from build123d import *

# Parameters (mm, degrees)
BOSS_EXTRUDE1_DEPTH      = 7.5
BOSS_EXTRUDE1_DEPTH_BACK = 7.5
SKETCH3_W                = 200
SKETCH3_H                = 15
CUT_EXTRUDE1_DEPTH       = 101.560926806
FILLET1_R                = 0.503257554
LPATTERN1_COUNT          = 42
LPATTERN1_PITCH          = 4.71238898
FILLET1_OF_LPATTERN1_R   = 0.503257554
CUT_EXTRUDE2_DEPTH       = 101.560926806
CUT_EXTRUDE2_DEPTH_BACK  = 101.560926806
SKETCH5_W                = 4.71238898
SKETCH5_H                = 3.375
CUT_EXTRUDE3_DEPTH       = 101.560926806
CUT_EXTRUDE3_DEPTH_BACK  = 101.560926806
SKETCH6_W                = 13.890612777
SKETCH6_H                = 21.950597968
CUT_EXTRUDE6_DEPTH       = 101.560926806
CUT_EXTRUDE6_DEPTH_BACK  = 101.560926806
SKETCH8_W                = 175.100830171
SKETCH8_H                = 44.946806771
SKETCH9_W                = 55.501850732
SKETCH9_H                = 10.784038355
CUT_EXTRUDE7_DEPTH       = 101.560926806
SKETCH10_W               = 10
SKETCH10_H               = 38
BOSS_EXTRUDE2_DEPTH      = 6.9
SKETCH11_W               = 12.54
SKETCH11_H               = 38
BOSS_EXTRUDE3_DEPTH      = 50
SKETCH12_W               = 2.54
SKETCH12_H               = 35
CUT_EXTRUDE8_DEPTH       = 121.701325593
CHAMFER1_SIZE            = 3
CHAMFER1_SIZE2           = 1.816762814
FILLET2_R                = 10
SKETCH13_W               = 39.144192087
SKETCH13_H               = 30
CUT_EXTRUDE9_DEPTH       = 5
CHAMFER2_SIZE            = 2
SKETCH14_R               = 1.5
CUT_EXTRUDE10_DEPTH      = 78.944675893


with BuildPart() as part:
    # Sketch3 → Boss-Extrude1 (new, two sides: drawn at the far end of the back side and taken through both)
    with BuildSketch(Plane.XY.offset(-BOSS_EXTRUDE1_DEPTH_BACK)):
        Rectangle(SKETCH3_W, SKETCH3_H)
    extrude(amount=BOSS_EXTRUDE1_DEPTH + BOSS_EXTRUDE1_DEPTH_BACK)

    # Sketch4 → Cut-Extrude1 (cut, symmetric)
    with BuildSketch(Plane.XY):
        Polygon((-94.247779608, 7.5), (-94.247779608, 4.125), (-94.743432664, 4.125), (-95.971832204, 7.5), align=None)
        Polygon((-97.236115992, 7.5), (-98.464515532, 4.125), (-98.960168588, 4.125), (-98.960168588, 7.5), align=None)
    cut_extrude1 = extrude(amount=CUT_EXTRUDE1_DEPTH, both=True, mode=Mode.SUBTRACT)

    # Fillet1
    fillet1_edges = [part.edges().sort_by_distance(p)[0] for p in [
        (-95.971832204, 7.5, 0),
        (-94.743432664, 4.125, 0),
        (-97.236115992, 7.5, 0),
        (-98.464515532, 4.125, 0),
    ]]
    fillet(fillet1_edges, radius=FILLET1_R)

    # LPattern1: Cut-Extrude1 ×42
    with Locations(*[(i * LPATTERN1_PITCH, 0, 0) for i in range(1, LPATTERN1_COUNT)]):
        add(cut_extrude1, mode=Mode.SUBTRACT)

    # Fillet1 of LPattern1
    fillet1_of_lpattern1_edges = [part.edges().sort_by_distance(p)[0] for p in [
        (-91.259443224, 7.5, 0),
        (-90.031043683, 4.125, 0),
        (-92.523727011, 7.5, 0),
        (-93.752126552, 4.125, 0),
        (-86.547054243, 7.5, 0),
        (-85.318654703, 4.125, 0),
        (-87.811338031, 7.5, 0),
        (-89.039737571, 4.125, 0),
        (-81.834665263, 7.5, 0),
        (-80.606265722, 4.125, 0),
        (-83.09894905, 7.5, 0),
        (-84.327348591, 4.125, 0),
        (-77.122276283, 7.5, 0),
        (-75.893876742, 4.125, 0),
        (-78.38656007, 7.5, 0),
        (-79.614959611, 4.125, 0),
        (-72.409887302, 7.5, 0),
        (-71.181487762, 4.125, 0),
        (-73.67417109, 7.5, 0),
        (-74.90257063, 4.125, 0),
        (-67.697498322, 7.5, 0),
        (-66.469098781, 4.125, 0),
        (-68.961782109, 7.5, 0),
        (-70.19018165, 4.125, 0),
        (-62.985109342, 7.5, 0),
        (-61.756709801, 4.125, 0),
        (-64.249393129, 7.5, 0),
        (-65.47779267, 4.125, 0),
        (-58.272720361, 7.5, 0),
        (-57.04432082, 4.125, 0),
        (-59.537004149, 7.5, 0),
        (-60.765403689, 4.125, 0),
        (-53.560331381, 7.5, 0),
        (-52.33193184, 4.125, 0),
        (-54.824615168, 7.5, 0),
        (-56.053014709, 4.125, 0),
        (-48.8479424, 7.5, 0),
        (-47.61954286, 4.125, 0),
        (-50.112226188, 7.5, 0),
        (-51.340625728, 4.125, 0),
        (-44.13555342, 7.5, 0),
        (-42.907153879, 4.125, 0),
        (-45.399837207, 7.5, 0),
        (-46.628236748, 4.125, 0),
        (-39.42316444, 7.5, 0),
        (-38.194764899, 4.125, 0),
        (-40.687448227, 7.5, 0),
        (-41.915847768, 4.125, 0),
        (-34.710775459, 7.5, 0),
        (-33.482375919, 4.125, 0),
        (-35.975059247, 7.5, 0),
        (-37.203458787, 4.125, 0),
        (-29.998386479, 7.5, 0),
        (-28.769986938, 4.125, 0),
        (-31.262670266, 7.5, 0),
        (-32.491069807, 4.125, 0),
        (-25.285997498, 7.5, 0),
        (-24.057597958, 4.125, 0),
        (-26.550281286, 7.5, 0),
        (-27.778680826, 4.125, 0),
        (-20.573608518, 7.5, 0),
        (-19.345208977, 4.125, 0),
        (-21.837892305, 7.5, 0),
        (-23.066291846, 4.125, 0),
        (-15.861219538, 7.5, 0),
        (-14.632819997, 4.125, 0),
        (-17.125503325, 7.5, 0),
        (-18.353902866, 4.125, 0),
        (-11.148830557, 7.5, 0),
        (-9.920431017, 4.125, 0),
        (-12.413114345, 7.5, 0),
        (-13.641513885, 4.125, 0),
        (-6.436441577, 7.5, 0),
        (-5.208042036, 4.125, 0),
        (-7.700725364, 7.5, 0),
        (-8.929124905, 4.125, 0),
        (-1.724052597, 7.5, 0),
        (-0.495653056, 4.125, 0),
        (-2.988336384, 7.5, 0),
        (-4.216735925, 4.125, 0),
        (2.988336384, 7.5, 0),
        (4.216735925, 4.125, 0),
        (1.724052596, 7.5, 0),
        (0.495653056, 4.125, 0),
        (7.700725364, 7.5, 0),
        (8.929124905, 4.125, 0),
        (6.436441577, 7.5, 0),
        (5.208042036, 4.125, 0),
        (12.413114345, 7.5, 0),
        (13.641513885, 4.125, 0),
        (11.148830557, 7.5, 0),
        (9.920431017, 4.125, 0),
        (17.125503325, 7.5, 0),
        (18.353902866, 4.125, 0),
        (15.861219538, 7.5, 0),
        (14.632819997, 4.125, 0),
        (21.837892305, 7.5, 0),
        (23.066291846, 4.125, 0),
        (20.573608518, 7.5, 0),
        (19.345208977, 4.125, 0),
        (26.550281286, 7.5, 0),
        (27.778680826, 4.125, 0),
        (25.285997498, 7.5, 0),
        (24.057597958, 4.125, 0),
        (31.262670266, 7.5, 0),
        (32.491069807, 4.125, 0),
        (29.998386479, 7.5, 0),
        (28.769986938, 4.125, 0),
        (35.975059247, 7.5, 0),
        (37.203458787, 4.125, 0),
        (34.710775459, 7.5, 0),
        (33.482375919, 4.125, 0),
        (40.687448227, 7.5, 0),
        (41.915847768, 4.125, 0),
        (39.42316444, 7.5, 0),
        (38.194764899, 4.125, 0),
        (45.399837207, 7.5, 0),
        (46.628236748, 4.125, 0),
        (44.13555342, 7.5, 0),
        (42.907153879, 4.125, 0),
        (50.112226188, 7.5, 0),
        (51.340625728, 4.125, 0),
        (48.8479424, 7.5, 0),
        (47.61954286, 4.125, 0),
        (54.824615168, 7.5, 0),
        (56.053014709, 4.125, 0),
        (53.560331381, 7.5, 0),
        (52.33193184, 4.125, 0),
        (59.537004148, 7.5, 0),
        (60.765403689, 4.125, 0),
        (58.272720361, 7.5, 0),
        (57.04432082, 4.125, 0),
        (64.249393129, 7.5, 0),
        (65.47779267, 4.125, 0),
        (62.985109341, 7.5, 0),
        (61.756709801, 4.125, 0),
        (68.961782109, 7.5, 0),
        (70.19018165, 4.125, 0),
        (67.697498322, 7.5, 0),
        (66.469098781, 4.125, 0),
        (73.67417109, 7.5, 0),
        (74.90257063, 4.125, 0),
        (72.409887302, 7.5, 0),
        (71.181487762, 4.125, 0),
        (78.38656007, 7.5, 0),
        (79.614959611, 4.125, 0),
        (77.122276283, 7.5, 0),
        (75.893876742, 4.125, 0),
        (83.09894905, 7.5, 0),
        (84.327348591, 4.125, 0),
        (81.834665263, 7.5, 0),
        (80.606265722, 4.125, 0),
        (87.811338031, 7.5, 0),
        (89.039737571, 4.125, 0),
        (86.547054243, 7.5, 0),
        (85.318654703, 4.125, 0),
        (92.523727011, 7.5, 0),
        (93.752126552, 4.125, 0),
        (91.259443224, 7.5, 0),
        (90.031043683, 4.125, 0),
        (97.236115992, 7.5, 0),
        (98.464515532, 4.125, 0),
        (95.971832204, 7.5, 0),
        (94.743432664, 4.125, 0),
    ]]
    fillet(fillet1_of_lpattern1_edges, radius=FILLET1_OF_LPATTERN1_R)

    # Sketch5 → Cut-Extrude2 (cut, two sides: drawn at the far end of the back side and taken through both)
    with BuildSketch(Plane.XY.offset(-CUT_EXTRUDE2_DEPTH_BACK)):
        with Locations((-101.316363078, 5.8125)):
            Rectangle(SKETCH5_W, SKETCH5_H)
        with Locations((101.316363078, 5.8125)):
            Rectangle(SKETCH5_W, SKETCH5_H)
    extrude(amount=CUT_EXTRUDE2_DEPTH + CUT_EXTRUDE2_DEPTH_BACK, mode=Mode.SUBTRACT)

    # Sketch6 → Cut-Extrude3 (cut, two sides: drawn at the far end of the back side and taken through both)
    with BuildSketch(Plane(origin=(0, 0, 0), x_dir=(0, 0, -1), z_dir=(1, 0, 0)).offset(-CUT_EXTRUDE3_DEPTH_BACK)):
        with Locations((5.945306389, -0.750264579)):
            Rectangle(SKETCH6_W, SKETCH6_H)
    extrude(amount=CUT_EXTRUDE3_DEPTH + CUT_EXTRUDE3_DEPTH_BACK, mode=Mode.SUBTRACT)

    # Sketch8 → Cut-Extrude6 (cut, two sides: drawn at the far end of the back side and taken through both)
    with BuildSketch(Plane.XY.offset(-CUT_EXTRUDE6_DEPTH_BACK)):
        with Locations((27.550415086, 7.242613414)):
            Rectangle(SKETCH8_W, SKETCH8_H)
    extrude(amount=CUT_EXTRUDE6_DEPTH + CUT_EXTRUDE6_DEPTH_BACK, mode=Mode.SUBTRACT)

    # Sketch9 → Cut-Extrude7 (cut, through all)
    with BuildSketch(Plane.XY):
        with Locations((-76.828993169, -6.642019178)):
            Rectangle(SKETCH9_W, SKETCH9_H)
    extrude(amount=CUT_EXTRUDE7_DEPTH, mode=Mode.SUBTRACT)

    # Sketch10 → Boss-Extrude2 (add)
    with BuildSketch(Plane(origin=(0, 0, 1), x_dir=(-1, 0, 0), z_dir=(0, 0, -1))):
        with Locations((65, 17.75)):
            Rectangle(SKETCH10_W, SKETCH10_H)
    extrude(amount=BOSS_EXTRUDE2_DEPTH)

    # Sketch11 → Boss-Extrude3 (add)
    with BuildSketch(Plane(origin=(0, 0, -5.9), x_dir=(-1, 0, 0), z_dir=(0, 0, -1))):
        with Locations((66.27, 17.75)):
            Rectangle(SKETCH11_W, SKETCH11_H)
    extrude(amount=BOSS_EXTRUDE3_DEPTH)

    # Sketch12 → Cut-Extrude8 (cut, through all)
    with BuildSketch(Plane.XZ.offset(1.25)):
        with Locations((-71.27, -23.4)):
            Rectangle(SKETCH12_W, SKETCH12_H)
        Polygon((-60, -5.9), (-63.8, -55.9), (-60, -55.9), align=None)
    extrude(amount=-CUT_EXTRUDE8_DEPTH, mode=Mode.SUBTRACT)

    # Chamfer1
    chamfer1_edges = [part.edges().sort_by_distance(p)[0] for p in [
        (-63.8, 17.75, -55.9),
    ]]
    chamfer1_side = [part.faces().sort_by_distance(p)[0] for p in [
        (-61.9, 17.75, -30.9),
    ]]
    chamfer(chamfer1_edges, length=CHAMFER1_SIZE, length2=CHAMFER1_SIZE2, reference=chamfer1_side[0])

    # Fillet2
    # the kernel refuses this fillet: 10 mm, written as the material it adds along each edge
    with BuildSketch(Plane(origin=(-70, -1.25, -40.9), x_dir=(-1, 0, 0), z_dir=(0, 1, 0))) as fillet2_piece_1:
        with BuildLine():
            CenterArc((10, 6.659459438), FILLET2_R, 180, 41.754936598)
            Line((0, 6.659459438), (-0.2, 6.659459438))
            Line((-0.2, 6.659459438), (-0.2, 0))
            Line((-0.2, 0), (0, -0.2))
            ThreePointArc((0, -0.2), (1.27, -0.2), (2.3908, -0.133189189))
            Line((2.3908, -0.133189189), (2.54, 0))
        make_face()
    extrude(amount=38)

    # Sketch13 → Cut-Extrude9 (cut)
    with BuildSketch(Plane(origin=(-59.20960532, 0, 4.499930004), x_dir=(-0.07578145826840343, 0, -0.997124450900044), z_dir=(0.997124450900044, 0, -0.07578145826840343))):
        with Locations((34.0020178, 17.75)):
            Rectangle(SKETCH13_W, SKETCH13_H)
    extrude(amount=-CUT_EXTRUDE9_DEPTH, mode=Mode.SUBTRACT)

    # Chamfer2
    chamfer2_edges = [part.edges().sort_by_distance(p)[0] for p in [
        (-62.79593696, 2.75, -9.699044158),
        (-62.79593696, 32.75, -9.699044158),
        (-65.762340919, 32.75, -48.730675198),
        (-65.762340919, 2.75, -48.730675198),
    ]]
    chamfer(chamfer2_edges, length=CHAMFER2_SIZE)

    # Sketch14 → Cut-Extrude10 (cut, through all)
    with BuildSketch(Plane(origin=(-60, 0, 0), x_dir=(0, 0, -1), z_dir=(1, 0, 0))):
        with Locations(Location((2.64, 27.75, 0), (0, 0, 90))):
            Circle(SKETCH14_R)
        with Locations(Location((2.64, 7.75, 0), (0, 0, 90))):
            Circle(SKETCH14_R)
    extrude(amount=-CUT_EXTRUDE10_DEPTH, mode=Mode.SUBTRACT)


solid = part.part
Part model, mm, in its own coordinate system. A direction names the side the tool comes from. Round coordinates to 2 decimals unless told otherwise and drop trailing zeros. Order: outer loops, then holes, each group sorted by start corner. A loop starts at its lowest first (then second) coordinate and runs counter-clockwise, first axis right, second up. Notation, with made-up numbers: (-21, -1.5) -> (29, -1.5) arc R9 ccw to (29, 8.5) -> close; hole circle Ø2 at (64, 72). An arc over 180 degrees is marked (long way). Put each result on its own line as item: value.
Q1. Band-saw the part on A-A (z = -2.64). Give the cut face in (x, y), and give its area (3 significant figures).
From the geometry:
outline: (-70, -1.25) -> (-60, -1.25) -> (-60, 6.25) -> (-70, 6.25) -> close; (-70, 9.25) -> (-60, 9.25) -> (-60, 26.25) -> (-70, 26.25) -> close; (-70, 29.25) -> (-60, 29.25) -> (-60, 36.75) -> (-70, 36.75) -> close
area: 320 mm2
Q2. Band-saw the part on D-D (z = -39). Give the cut face in (x, y), and give its area (3 significant figures).
From the geometry:
outline: (-71.21, -1.25) -> (-62.52, -1.25) -> (-62.52, 2.75) -> (-67.53, 2.75) -> (-67.53, 32.75) -> (-62.52, 32.75) -> (-62.52, 36.75) -> (-71.21, 36.75) -> close
area: 180 mm2
Q3. Band-saw the part on B-B (y = 27). Give the cut face in (x, z), and give its area (3 significant figures).
From the geometry:
outline: (-72.54, -55.9) -> (-65.62, -55.9) -> (-63.57, -52.91) -> (-63.27, -48.92) -> (-68.26, -48.54) -> (-65.29, -9.51) -> (-60.3, -9.89) -> (-60, -5.9) -> (-60, -3.94) -> (-70, -3.94) -> (-70, -34.24) arc R10 cw to (-72.54, -40.9) -> close; (-70, -1.34) -> (-60, -1.34) -> (-60, 1) -> (-70, 1) -> close
area: 293 mm2
Q4. Wall check: line 1 (Z direction, x = -64.75, y = 27.75); line 2 (Y direction, x = -63, z = -2); line 3 (Y direction, x = -63.5, z = -37). Give the ranges that are in metal, low to high. Write a range as [from, to].
From the geometry:
line 1: z = [-54.63, -48.81], [-9.55, -4.14], [-1.14, 1]
line 2: y = [-1.25, 6.39], [9.11, 26.39], [29.11, 36.75]
line 3: y = [-1.25, 2.75], [32.75, 36.75]
Q5. Band-saw the part on C-C (y = 12.5). Give the cut face in (x, z).
From the geometry:
outline: (-72.54, -55.9) -> (-65.62, -55.9) -> (-63.57, -52.91) -> (-63.27, -48.92) -> (-68.26, -48.54) -> (-65.29, -9.51) -> (-60.3, -9.89) -> (-60, -5.9) -> (-60, 1) -> (-70, 1) -> (-70, -34.24) arc R10 cw to (-72.54, -40.9) -> close
Q6. Pin check, flat tips, straight feed: pin 1 Ø9.5 at (x, y) = (-92, 5) entering from -Z; pin 2 Ø4 at (x, y) = (-73, 17) entering from +Z; pin 3 Ø0.6 at (x, z) = (-92, 3) entering from +Y. Stop position of each tip, or through.
From the geometry:
pin 1: stops at z = 1
pin 2: stops at z = -38.6
pin 3: stops at y = 7.5
Q7. Tool access for faces 1 (the face through (-72.54, 17, -48)), 2 (the face through (-62.84, 31.76, -10.71)), 3 (the face through (-64, 32.75, -29)), 4 (the face through (-86, 6, 4)), 5 (the face through (-64.857, 5.831, 4.295)): list every direction of +Z, -Z, +X, -X, +Y, -Y with a clear straight run to the whole face (end or side of a thin tool).
From the geometry:
face 1: -Z, -X, +Y, -Y
face 2: none
face 3: +X
face 4: +Z, -Z, +Y
face 5: +Z, +Y
Q8. Pull direction X, two halves, no side cores. Call faces 6 (the face through (-80, 2, 7.5)), 7 (the face through (-70, 17, -16)), 8 (the face through (-93.13, 5.83, 4.3)), 9 (the face through (-60.3, 5.4, 4.3)): pulls with the +X half, pulls with the -X half, needs draft (parallel to the pull), parting line crosses it, or undercut.
From the geometry:
face 6: needs draft
face 7: pulls with the -X half
face 8: undercut
face 9: undercut
